Part model, mm, in its own coordinate system. Face numbers are marked on the shaded views. A direction names the side the tool comes from. Round coordinates to 2 decimals unless told otherwise and drop trailing zeros. Loops run counter-clockwise (first coordinate to the right, second up) from the corner with the lowest first, then second, coordinate; pieces in that order, holes last. Notation, with made-up numbers: M 87,36 L 112,36 A12 ccw 112,44 Z; hole C 64.5,71.5 d3. An arc over 180 degrees is marked long. Put each result on its own line as item: value. Start each with the question number.
1) Slice it at B-B on z = -19. Give the cut face in (x, y).
2) Drop flat-ended pins along their axis: pin 1 Ø1.5 at (y, z) = (1, -17.5) entering from +X; pin 2 Ø3 at (x, z) = (2.5, -2.5) entering from +Y; pin 3 Ø4 at (y, z) = (0, -11.5) entering from -X. Give the stop position or say it passes through.
3) Slice it at D-D on x = -2.5. Give the cut face in (y, z).
4) Probe line 1 along Z through (x, y) = (0.5, -2.25); line 2 along X through (y, z) = (0, -15.25); line 3 along Z through (x, y) = (1.5, 1.25). List the from-to ranges inside material, lowest first.
5) Which spindle directions (+Z, -Z, +X, -X, +Y, -Y) get a long thin tool onto all of the face, cutting with end or side? Do the marked faces 1 and 2. Say none if no direction does.
Solid Edge part; units mm, degrees
sketch "Sketch1" plane through (0, 0, 0) normal (0, 0, 1) x (1, 0, 0)
  circle A0 centre (0, 0) radius 4.06
extrude "Protrusion1" add sketch "Sketch1" along normal blind 3
sketch "Sketch2" plane through (0, 0, 0) normal (0, 0, -1) x (1, 0, 0)
  circle A0 centre (0, 0) radius 2
extrude "Protrusion2" add sketch "Sketch2" along normal blind 25
sketch "Sketch3" plane through (0, 0, -25) normal (0, 0, -1) x (1, 0, 0)
  circle A0 centre (0, 0) radius 1.9997
extrude "Cutout1" cut sketch "Sketch3" against normal blind 14 flip side to cut
chamfer "Chamfer_1" distance 0.3 angle 45 1 edges at (-1.9997, 0, -25)
sketch "Sketch4" plane through (0, 0, 3) normal (0, 0, 1) x (1, 0, 0)
  line L0 (-2.0576, 3.5) -> (2.0576, 3.5)
extrude "Cutout2" cut sketch "Sketch4" against normal up to next material side at (0, 3.55, 3)
pattern_circular "Pattern1" count 6 over 360 about axis through (0, 0, 3) along (0, 0, 1) of "Cutout2"
properties part number "215862" material "Stainless Steel, 304"
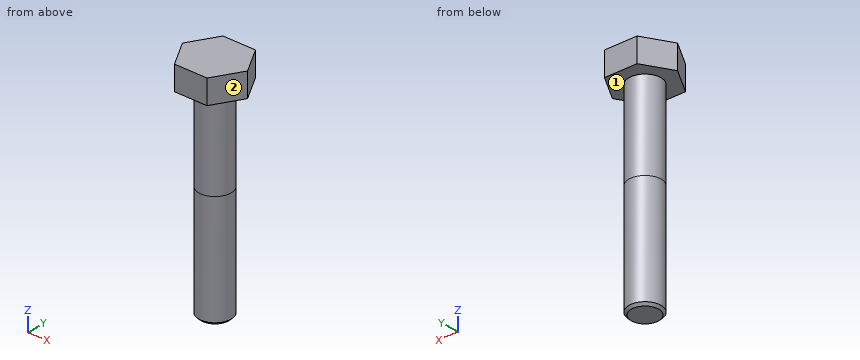
Recorded:
1. outline: C 0,0 d4
2. pin 1: stops at x = 1.98
2. pin 2: stops at y = 1.73
2. pin 3: stops at x = -2
3. outline: M -2.67,0 L 2.67,0 L 2.67,3 L -2.67,3 Z
4. line 1: z = 0 to 3
4. line 2: x = -2 to 2
4. line 3: z = -24.75 to 3
5. face 1: -Z
5. face 2: +Z, -Z, +X, -Y
